from build123d import *

# Parameters (mm, degrees)
CROQUIS1_R              = 3
SALIENTE_EXTRUIR1_DEPTH = 73.5
REDONDEO1_R             = 0.25
SKETCH1_W               = 3.065124184
SKETCH1_H               = 10
CUT_EXTRUDE1_DEPTH      = 12


with BuildPart() as part:
    # Croquis1 → Saliente-Extruir1 (new body)
    with BuildSketch(Plane.XY):
        Circle(CROQUIS1_R)
    extrude(amount=SALIENTE_EXTRUIR1_DEPTH)

    # Redondeo1
    redondeo1_edges = [part.edges().sort_by_distance(p)[0] for p in [
        (-3, 0, 73.5),
    ]]
    fillet(redondeo1_edges, radius=REDONDEO1_R)

    # Sketch1 → Cut-Extrude1 (cut)
    with BuildSketch(Plane.XY.offset(73.5)):
        with Locations((3.332562092, 1.320530023)):
            Rectangle(SKETCH1_W, SKETCH1_H)
    extrude(amount=-CUT_EXTRUDE1_DEPTH, mode=Mode.SUBTRACT)


solid = part.part
Can you work these out from the model? Positions are in its coordinate system, mm. A direction names the side the tool comes from. Round coordinates to 2 decimals unless told otherwise and drop trailing zeros. Order: outer loops, then holes, each group sorted by start corner. A loop starts at its lowest first (then second) coordinate and runs counter-clockwise, first axis right, second up. Notation, with made-up numbers: (8, 71) -> (65, 71) arc R16 ccw to (65, 96) -> close; hole circle Ø2 at (10, -9). An arc over 180 degrees is marked (long way). Write each question's results on one line, items separated by ' | '. Start each with the question number.
Item 1: If we section it at C-C, the plane z = 62.5: Write out the boundary of the cut face in (x, y).
Item 2: If we section it at B-B, the plane z = 41: Write out the boundary of the cut face in (x, y), then the cut area to 3 significant figures.
Item 3: If we section it at A-A, the plane y = 0: Write out the boundary of the cut face in (x, z).
Item 4: Which directions (+Z, -Z, +X, -X, +Y, -Y) give clear straight access to the entire face, cutting with the end or side of a thin tool? Please do faces 1 (the cylindrical face through (-3, 0, 36)), 2 (the flat face through (1.8, 0, 68)).
Item 5: Will these pins go through, and if not, where does the flat tip stop? pin 1 (2.5 mm diameter, centred on y = 0, z = 70, fed in from +X); pin 2 (1.3 mm diameter, centred on x = 2.5, y = 1, fed in from +Z).
Item 6: Please list where these lines run through material, in increasing order: L1, parallel to Z at x = 2, y = -1; L2, parallel to Y at x = 0.5, z = 16.5; L3, parallel to X at y = 2, z = 53.
Results:
1) outline: (1.8, -2.4) -> (1.8, 2.4) arc R3 ccw (long way) to start
2) outline: circle Ø6 at (0, 0) | area: 28.3 mm2
3) outline: (-3, 0) -> (3, 0) -> (3, 61.5) -> (1.8, 61.5) -> (1.8, 73.5) -> (-2.75, 73.5) arc R0.25 ccw to (-3, 73.25) -> close
4) face 1: +Z, -Z | face 2: +Z, +X, +Y, -Y
5) pin 1: stops at x = 1.8 | pin 2: stops at z = 61.5
6) L1: z = 0 to 61.5 | L2: y = -2.96 to 2.96 | L3: x = -2.24 to 2.24
